```python
from build123d import *

# Parameters (mm, degrees)
SKETCH1_R           = 1
BOSS_EXTRUDE1_DEPTH = 4


with BuildPart() as part:
    # Sketch1 → Boss-Extrude1 (new body)
    with BuildSketch(Plane.XY):
        with BuildLine():
            Line((0, 0), (-5, 0))
            ThreePointArc((-5, 0), (-15.606601718, -4.393398282), (-20, -15))
            Line((-20, -15), (-20, -31))
            ThreePointArc((-20, -31), (-19.414213562, -32.414213562), (-18, -33))
            Line((-18, -33), (-1.488039242, -28.627581694))
            ThreePointArc((-1.488039242, -28.627581694), (-0.415083359, -27.914069878), (0, -26.694217739))
            Line((0, -26.694217739), (0, 0))
        make_face()
        with Locations((-18.5, -31)):
            Circle(SKETCH1_R, mode=Mode.SUBTRACT)
        with Locations((-2, -25.628432728)):
            Circle(SKETCH1_R, mode=Mode.SUBTRACT)
    extrude(amount=BOSS_EXTRUDE1_DEPTH)


solid = part.part
```
Check sheet for the modelled part. Datum: model origin and axes. Units: mm. Round coordinates to 2 decimals unless told otherwise and drop trailing zeros. Write each loop counter-clockwise with the first axis right and the second up, starting at its lowest first coordinate (ties: lowest second). Pieces come first, ordered by that corner, then holes. Notation, with made-up numbers: M 72.5,18 L 83.5,18 A20 cw 83.5,38 Z; hole C 72.5,17 d11. An arc over 180 degrees is marked long. Write item = value, one per line. Start each with the question number.
1. Section check D-D, the plane y = -3.5. Record the cut outline in (x, z), then the cut area to 3 significant figures.
2. Section check A-A, the plane x = -2. Record the cut outline in (y, z), then the cut area to 3 significant figures.
3. Gauge pin test, flat ends, axial feed: pin 1 (1.5 mm diameter, centred on y = -4.5, z = 1.5, fed in from -X); pin 2 (1.8 mm diameter, centred on x = -18.5, y = -31, fed in from -Z). Record the tip position at first contact, or that the pin passes through.
4. Section check B-B, the plane z = 3.25. Record the cut outline in (x, y), then the cut area to 3 significant figures.
5. Section check C-C, the plane x = -18.5. Record the cut outline in (y, z).
6. Scan lines: line 1 (Y direction, x = -2, z = 2.55); line 2 (Y direction, x = -18.5, z = 1.35); line 3 (Y direction, x = -9.5, z = 1.1). Record each from-to range of solid material in increasing order. Write a range as [from, to].
7. Release check for a two-part mould opening along Y. For faces 1 (the cylindrical face through (-18.63, -30.01, 1.97)), 2 (the flat face through (0, -14, 2)), 3 (the cylindrical face through (-0.43, -27.93, 1.97)), 4 (the flat face through (-2, 0, 2)) record: pulls with the +Y half, pulls with the -Y half, needs draft (parallel to the pull), parting line crosses it, or undercut.
Results found:
q1.outline = M -14.63,0 L 0,0 L 0,4 L -14.63,4 Z
q1.area = 58.5 mm^2
q2.outline = M -28.76,0 L -26.63,0 L -26.63,4 L -28.76,4 Z; M -24.63,0 L 0,0 L 0,4 L -24.63,4 Z
q2.area = 107 mm^2
q3.pin_1 = -16.4
q3.pin_2 = through
q4.outline = M -20,-31 A2 ccw -18,-33 L -1.49,-28.63 A2 ccw 0,-26.69 L 0,0 L -5,0 A15 ccw -20,-15 Z; hole C -18.5,-31 d2; hole C -2,-25.63 d2
q4.area = 561 mm^2
q5.outline = M -32.94,0 L -32,0 L -32,4 L -32.94,4 Z; M -30,0 L -8.46,0 L -8.46,4 L -30,4 Z
q6.line_1 = [-28.76, -26.63], [-24.63, 0]
q6.line_2 = [-32.94, -32], [-30, -8.46]
q6.line_3 = [-30.75, -0.69]
q7.face_1 = undercut
q7.face_2 = needs draft
q7.face_3 = pulls with the -Y half
q7.face_4 = pulls with the +Y half
